Answer from the drawing. Dimensions are ordinates in mm from the lowest x, y and z of the part. Round coordinates to 2 decimals unless told otherwise and drop trailing zeros. Loops run counter-clockwise (first coordinate to the right, second up) from the corner with the lowest first, then second, coordinate; pieces in that order, holes last. Notation, with made-up numbers: M 60.25,40 L 84.25,40 A21 ccw 84.25,69 Z; hole C 20,-24.75 d1. An arc over 180 degrees is marked long. Answer as a JSON object with one key per item and string values.
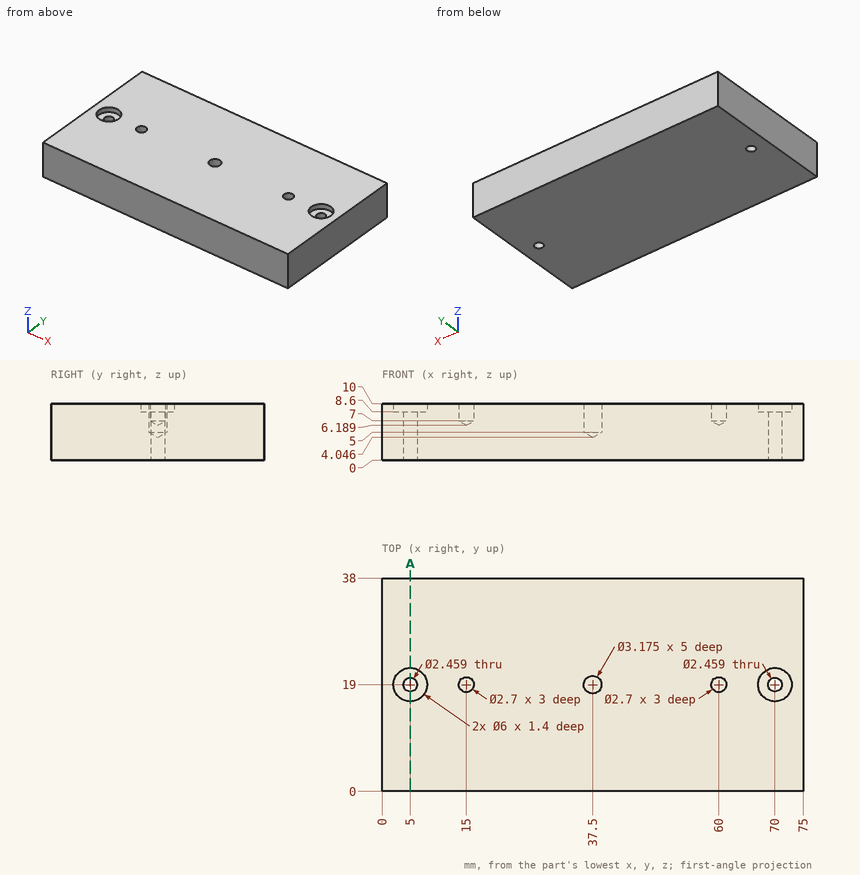
Item 1: A flat-ended cylindrical pin translates along its axis: P1, Ø5, axis at x = 5, y = 19, coming from the +Z side. Find the tip coordinate at first contact, or state that the pin passes through.
Values follow:
{"P1": "z = 8.6"}
Item 2: The part is cut by section A-A (x = 5). Give the vertices of the cut face in (y, z).
Values follow:
{"outline": "M 0,0 L 17.77,0 L 17.77,8.6 L 16,8.6 L 16,10 L 0,10 Z; M 20.23,0 L 38,0 L 38,10 L 22,10 L 22,8.6 L 20.23,8.6 Z"}
Item 3: Straight lines are drawn through the part: line 1 (X direction, y = 19, z = 7.7); line 2 (X direction, y = 19, z = 5); line 3 (Y direction, x = 5, z = 9.4). For each, find the intervals that lie inside material, in ascending order.
Values follow:
{"line 1": "0 to 3.77, 6.23 to 13.65, 16.35 to 35.91, 39.09 to 58.65, 61.35 to 68.77, 71.23 to 75", "line 2": "0 to 3.77, 6.23 to 35.91, 39.09 to 68.77, 71.23 to 75", "line 3": "0 to 16, 22 to 38"}
